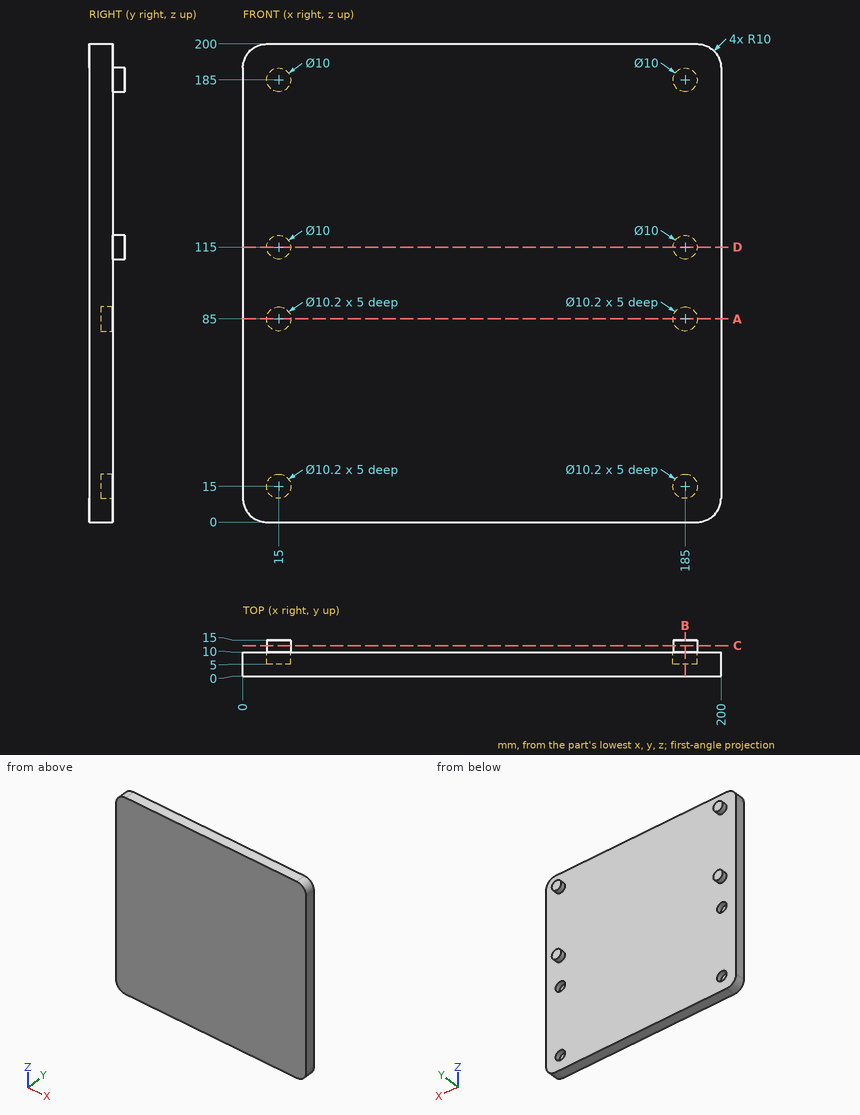
Geometry: see drawing. Coordinates: mm, zero at the bounding-box minimum. Round coordinates to 2 decimals unless told otherwise and drop trailing zeros. Write each loop counter-clockwise with the first axis right and the second up, starting at its lowest first coordinate (ties: lowest second). Pieces come first, ordered by that corner, then holes. Notation, with made-up numbers: M 59,-12 L 69,-12 A16 ccw 69,-7 Z; hole C 27,-11 d9. An arc over 180 degrees is marked long. Answer as a JSON object with one key per item and string values. Group by question number.
(1) Ray query, line 1 (X direction, y = 7.65, z = 15); line 2 (Y direction, x = 151, z = 143.5); line 3 (Z direction, x = 11, y = 11.5). Return the intervals inside material, ascending. Write a range as [from, to].
(2) First-contact query: pin 1 (6 mm diameter, centred on x = 79, z = 110.5, fed in from +Y); pin 2 (8 mm diameter, centred on x = 185, z = 85, fed in from -Y); pin 3 (3 mm diameter, centred on x = 15.5, z = 16, fed in from +Y). Flat tips, straight axial feed; report the tip coordinate or a pass-through.
(3) Section query B-B on x = 185. Output: boundary loops of the cut face in (y, z), then the cut area to 3 significant figures.
(4) Section query A-A on z = 85. Output: boundary loops of the cut face in (x, y), then the cut area to 3 significant figures.
(5) Section query D-D on z = 115. Output: boundary loops of the cut face in (x, y).
(6) Section query C-C on y = 12.75. Output: boundary loops of the cut face in (x, z), then the cut area to 3 significant figures.
Computed values:
{
 "1": {"line 1": "[0, 9.9], [20.1, 179.9], [190.1, 200]", "line 2": "[0, 10]", "line 3": "[112, 118], [182, 188]"},
 "2": {"pin 1": "y = 10", "pin 2": "y = 0", "pin 3": "y = 5"},
 "3": {"outline": "M 0,0 L 10,0 L 10,9.9 L 5,9.9 L 5,20.1 L 10,20.1 L 10,79.9 L 5,79.9 L 5,90.1 L 10,90.1 L 10,110 L 15,110 L 15,120 L 10,120 L 10,180 L 15,180 L 15,190 L 10,190 L 10,200 L 0,200 Z", "area": "2,000 mm^2"},
 "4": {"outline": "M 0,0 L 200,0 L 200,10 L 190.1,10 L 190.1,5 L 179.9,5 L 179.9,10 L 20.1,10 L 20.1,5 L 9.9,5 L 9.9,10 L 0,10 Z", "area": "1,900 mm^2"},
 "5": {"outline": "M 0,0 L 200,0 L 200,10 L 190,10 L 190,15 L 180,15 L 180,10 L 20,10 L 20,15 L 10,15 L 10,10 L 0,10 Z"},
 "6": {"outline": "C 15,115 d10; C 15,185 d10; C 185,115 d10; C 185,185 d10", "area": "314 mm^2"}
}
